Source: three-view drawing plus pictorial views. Frame: mm from the lowest corner of the part. Coordinates: 2 decimals unless noted, no trailing zeros. Write each loop counter-clockwise with the first axis right and the second up, starting at its lowest first coordinate (ties: lowest second). Pieces come first, ordered by that corner, then holes. Notation, with made-up numbers: M -30.5,68 L -13.5,68 A20 cw -13.5,75 Z; hole C -11,2 d7. An arc over 180 degrees is marked long. Write item = value, one per line. Start each with the question number.
Item 1: Section C-C on x = 53. Output: boundary loops of the cut face in (y, z).
Item 2: Section B-B on z = 21. Output: boundary loops of the cut face in (x, y).
Item 3: Ray query, L1, parallel to X at y = 1.4, z = 74 (1 decimal); L2, parallel to X at y = 0.4, z = 16.5 (1 decimal); L3, parallel to Z at x = 44, y = 1.6. Return the intervals inside material, ascending. Write a range as [from, to].
Item 4: Section A-A on y = 1.35. Output: boundary loops of the cut face in (x, z), plus the area to 3 significant figures.
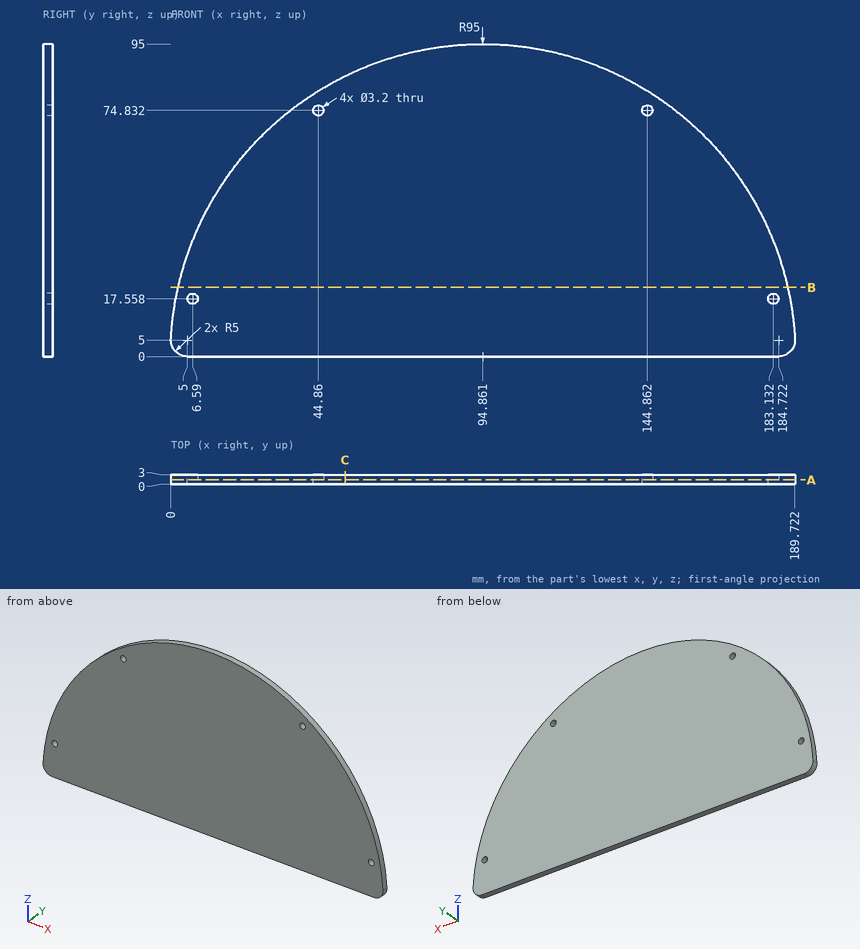
Responses:
q1.outline = M 0,0 L 3,0 L 3,85.28 L 0,85.28 Z
q2.outline = M 2.21,0 L 187.51,0 L 187.51,3 L 2.21,3 Z
q3.L1 = [35.3, 43.5], [46.2, 143.5], [146.2, 154.4]
q3.L2 = [1.3, 5.4], [7.8, 181.9], [184.3, 188.4]
q3.L3 = [0, 73.48], [76.18, 80.24]
q4.outline = M 0.01,5.28 A5 ccw 5,0 L 184.72,0 A5 ccw 189.71,5.28 A95 ccw Z; hole C 6.59,17.56 d3.2; hole C 44.86,74.83 d3.2; hole C 144.86,74.83 d3.2; hole C 183.13,17.56 d3.2
q4.area = 14,100 mm²
